Work out the finished part from the listing and answer in its coordinate system (mm). A direction names the side the tool comes from. Coordinates: 2 decimals unless noted, no trailing zeros. Use a Markdown table: item, result.
from build123d import *

# Parameters (mm, degrees)
BOSS_EXTRUDE1_DEPTH = 30
CHAMFER1_SIZE       = 13.5
FILLET1_R           = 50
FILLET2_R           = 50
SHELL1_T            = -5
CUT_EXTRUDE1_REACH  = 183.384
SKETCH5_W           = 85.5
SKETCH5_H           = 65.5
CUT_EXTRUDE2_DEPTH  = 2
SKETCH6_R           = 10.1203125
CUT_EXTRUDE3_DEPTH  = 1.488
CUT_EXTRUDE4_START  = -1.488
SKETCH7_R           = 10.1203125
CUT_EXTRUDE4_DEPTH  = 1.488
CUT_EXTRUDE5_REACH  = 198.109
SKETCH8_R           = 7.9375
BOSS_EXTRUDE2_START = -25
BOSS_EXTRUDE2_DEPTH = 22.5
CUT_EXTRUDE6_START  = -2.5
CUT_EXTRUDE6_DEPTH  = 5
SKETCH11_R          = 2.1
CUT_EXTRUDE7_DEPTH  = 155.677082983
CUT_EXTRUDE8_REACH  = 210.327
SKETCH12_R          = 8.1


with BuildPart() as part:
    # Sketch3 → Boss-Extrude1 (new body)
    with BuildSketch(Plane(origin=(0, 0, 0), x_dir=(1, 0, 0), z_dir=(0, 1, 0))):
        Polygon((80, 0), (80, -100), (30, -130), (-30, -130), (-80, -100), (-80, 0), (-30, 30), (30, 30), align=None)
    extrude(amount=BOSS_EXTRUDE1_DEPTH)

    # Chamfer1
    chamfer1_edges = [part.edges().sort_by_distance(p)[0] for p in [
        (-55, 30, 115),
        (0, 30, 130),
        (55, 30, 115),
    ]]
    chamfer(chamfer1_edges, length=CHAMFER1_SIZE)

    # Fillet1
    # the kernel refuses this fillet: 50 mm, written as the material it takes off along each edge
    with BuildSketch(Plane(origin=(30, -34.622995619, 130), x_dir=(0.857492925712544, 0, -0.5144957554275268), z_dir=(0, 1, 0)), Plane(origin=(-30, -34.622995619, 130), x_dir=(1, 0, 0), z_dir=(0, 1, 0))) as fillet1_piece_1:
        with BuildLine():
            CenterArc((FILLET1_R * 0.276983964948, FILLET1_R), FILLET1_R, 239.036243468, 30.963756532)
            Line((-FILLET1_R * 0.237511790479, FILLET1_R * 0.142507074287), (0, 0))
            Line((0, 0), (FILLET1_R * 0.276983964948, 0))
        make_face()
    extrude(amount=85.745991237, mode=Mode.SUBTRACT)
    with BuildSketch(Plane(origin=(-80, -39.074271729, 164.810181009), x_dir=(0, -0.759125277171481, -0.6509445549041194), z_dir=(0, 0.6509445549041194, -0.759125277171481))) as fillet1_piece_2:
        with BuildLine():
            CenterArc((FILLET1_R * 0.682998529574, -FILLET1_R), FILLET1_R, 90, 68.666037253)
            Line((-FILLET1_R * 0.248477212904, -FILLET1_R * 0.636196562446), (0, 0))
            Line((0, 0), (FILLET1_R * 0.682998529574, 0))
        make_face()
    extrude(amount=191.488725913, mode=Mode.SUBTRACT)
    with BuildSketch(Plane(origin=(80, -39.074271729, 164.810181009), x_dir=(0, -0.759125277171481, -0.6509445549041195), z_dir=(0, 0.6509445549041195, -0.759125277171481))) as fillet1_piece_3:
        with BuildLine():
            CenterArc((FILLET1_R * 0.682998529574, FILLET1_R), FILLET1_R, 201.333962747, 68.666037253)
            Line((-FILLET1_R * 0.248477212904, FILLET1_R * 0.636196562446), (0, 0))
            Line((0, 0), (FILLET1_R * 0.682998529574, 0))
        make_face()
    extrude(amount=191.488725913, mode=Mode.SUBTRACT)
    with BuildSketch(Plane(origin=(34.617865704, -0.171960433, 146.671960433), x_dir=(0.9114297192816029, -0.13590975982943138, -0.3883611772478869), z_dir=(-0.19220542560964893, 0.6939225729021263, -0.6939225729021263)), Plane(origin=(-34.617865704, -0.171960433, 146.671960433), x_dir=(0.9813547138350198, -0.13590975982942916, 0.13590975982942954), z_dir=(0.19220542560964907, 0.6939225729021263, -0.6939225729021263))) as fillet1_piece_4:
        with BuildLine():
            CenterArc((FILLET1_R * 0.19220542561, FILLET1_R), FILLET1_R, 248.24024707, 21.75975293)
            Line((-FILLET1_R * 0.178510109177, FILLET1_R * 0.0712535371437), (0, 0))
            Line((0, 0), (FILLET1_R * 0.19220542561, 0))
        make_face()
    extrude(amount=67.505976453, mode=Mode.SUBTRACT)

    # Fillet2
    fillet2_edges = [part.edges().sort_by_distance(p)[0] for p in [
        (30, 15, -30),
        (-30, 15, -30),
    ]]
    fillet(fillet2_edges, radius=FILLET2_R)

    # Shell1
    shell1_openings = [part.faces().sort_by_distance(p)[0] for p in [
        (0, 30, 41.507073617),
    ]]
    offset(amount=SHELL1_T, openings=shell1_openings)

    # Sketch4 → Cut-Extrude1 (cut, up to next)
    with BuildSketch(Plane.XY.offset(130), mode=Mode.PRIVATE) as cut_extrude1_sk1:
        Polygon((10.55, 13.832263561), (10.55, 8.567736439), (6.776999518, 6), (-10.55, 6), (-10.55, 16.4), (6.776999518, 16.4), align=None)
    cut_extrude1_tool1 = extrude(cut_extrude1_sk1.sketch, amount=-CUT_EXTRUDE1_REACH, mode=Mode.PRIVATE) & part.part
    add(cut_extrude1_tool1.solids().sort_by_distance((-0.429196, 11.2, 130))[0], mode=Mode.SUBTRACT)

    # Sketch5 → Cut-Extrude2 (cut)
    with BuildSketch(Plane(origin=(0, 5, 0), x_dir=(1, 0, 0), z_dir=(0, 1, 0))):
        with Locations((-7.25, -42.75)):
            Rectangle(SKETCH5_W, SKETCH5_H)
    extrude(amount=-CUT_EXTRUDE2_DEPTH, mode=Mode.SUBTRACT)

    # Sketch6 → Cut-Extrude3 (cut)
    with BuildSketch(Plane(origin=(21.176470588, 0, -35.294117647), x_dir=(-0.8574929257125442, 0, -0.5144957554275265), z_dir=(0.5144957554275265, 0, -0.8574929257125442))):
        with Locations((-39.259425856, 15.1203125)):
            Circle(SKETCH6_R)
    cut_extrude3 = extrude(amount=-CUT_EXTRUDE3_DEPTH, mode=Mode.SUBTRACT)

    # Sketch7 → Cut-Extrude4 (cut)
    with BuildSketch(Plane(origin=(18.603991811, 0, -31.006653018), x_dir=(0.8574929257125442, 0, 0.5144957554275265), z_dir=(-0.5144957554275265, 0, 0.8574929257125442)).offset(CUT_EXTRUDE4_START)):
        with Locations(Location((39.259425856, 15.1203125, 0), (0, 0, 180))):
            Circle(SKETCH7_R)
    cut_extrude4 = extrude(amount=CUT_EXTRUDE4_DEPTH, mode=Mode.SUBTRACT)

    # Sketch8 → Cut-Extrude5 (cut, up to next)
    with BuildSketch(Plane(origin=(21.176470588, 0, -35.294117647), x_dir=(-0.8574929257125442, 0, -0.5144957554275265), z_dir=(0.5144957554275265, 0, -0.8574929257125442)), mode=Mode.PRIVATE) as cut_extrude5_sk1:
        with Locations((-39.259425856, 15.1203125)):
            Circle(SKETCH8_R)
    cut_extrude5_tool1 = extrude(cut_extrude5_sk1.sketch, amount=-CUT_EXTRUDE5_REACH, mode=Mode.PRIVATE) & part.part
    cut_extrude5 = cut_extrude5_tool1.solids().sort_by_distance((54.841151, 15.120313, -15.09531))[0]
    add(cut_extrude5, mode=Mode.SUBTRACT)

    # Mirror1: Cut-Extrude3, Cut-Extrude4, Cut-Extrude5 across plane
    add(cut_extrude3.mirror(Plane(origin=(0, 0, 0), x_dir=(0, 0, 1), z_dir=(1, 0, 0))), mode=Mode.SUBTRACT)
    add(cut_extrude4.mirror(Plane(origin=(0, 0, 0), x_dir=(0, 0, 1), z_dir=(1, 0, 0))), mode=Mode.SUBTRACT)
    add(cut_extrude5.mirror(Plane(origin=(0, 0, 0), x_dir=(0, 0, 1), z_dir=(1, 0, 0))), mode=Mode.SUBTRACT)

    # Sketch9 → Boss-Extrude2 (add)
    with BuildSketch(Plane(origin=(0, 30, 0), x_dir=(1, 0, 0), z_dir=(0, 1, 0)).offset(BOSS_EXTRUDE2_START)):
        with BuildLine():
            Line((-75, -2.830951895), (-66.425070743, 2.314005659))
            Line((-66.425070743, 2.314005659), (-62.074071209, -0.149488415))
            ThreePointArc((-62.074071209, -0.149488415), (-58.789057061, -12.009431821), (-70.649000466, -15.29444597))
            Line((-70.649000466, -15.29444597), (-75, -12.830951895))
            Line((-75, -12.830951895), (-75, -2.830951895))
        make_face()
    boss_extrude2 = extrude(amount=BOSS_EXTRUDE2_DEPTH)

    # Sketch10 → Cut-Extrude6 (cut)
    with BuildSketch(Plane(origin=(0, 30, 0), x_dir=(1, 0, 0), z_dir=(0, 1, 0)).offset(CUT_EXTRUDE6_START)):
        Polygon((-62.361535838, -5.412566116), (-66.361535838, -3.103165039), (-70.361535838, -5.412566116), (-70.361535838, -10.031368269), (-66.361535838, -12.340769346), (-62.361535838, -10.031368269), align=None)
    cut_extrude6 = extrude(amount=-CUT_EXTRUDE6_DEPTH, mode=Mode.SUBTRACT)

    # Mirror2: Boss-Extrude2, Cut-Extrude6 across plane
    add(boss_extrude2.mirror(Plane(origin=(0, 0, 0), x_dir=(0, 0, 1), z_dir=(1, 0, 0))))
    add(cut_extrude6.mirror(Plane(origin=(0, 0, 0), x_dir=(0, 0, 1), z_dir=(1, 0, 0))), mode=Mode.SUBTRACT)

    # Sketch11 → Cut-Extrude7 (cut, through all)
    with BuildSketch(Plane(origin=(0, 5, 0), x_dir=(1, 0, 0), z_dir=(0, 1, 0))):
        with Locations(Location((-27.25, -95.5, 0), (0, 0, 270))):
            Circle(SKETCH11_R)
        with Locations(Location((-20, 19, 0), (0, 0, 270))):
            Circle(SKETCH11_R)
    cut_extrude7 = extrude(amount=-CUT_EXTRUDE7_DEPTH, mode=Mode.SUBTRACT)

    # Mirror3: Cut-Extrude7 across plane
    add(cut_extrude7.mirror(Plane(origin=(0, 0, 0), x_dir=(0, 0, 1), z_dir=(1, 0, 0))), mode=Mode.SUBTRACT)

    # Sketch12 → Cut-Extrude8 (cut, up to next)
    with BuildSketch(Plane(origin=(80, 0, 0), x_dir=(0, 0, -1), z_dir=(1, 0, 0)), mode=Mode.PRIVATE) as cut_extrude8_sk1:
        with Locations((-32.830951895, 16.25)):
            Circle(SKETCH12_R)
    cut_extrude8_tool1 = extrude(cut_extrude8_sk1.sketch, amount=-CUT_EXTRUDE8_REACH, mode=Mode.PRIVATE) & part.part
    add(cut_extrude8_tool1.solids().sort_by_distance((80, 16.25, 32.830952))[0], mode=Mode.SUBTRACT)


solid = part.part
Q1. Consider line 1 (X direction, y = 6.5, z = 39.5); line 2 (Z direction, x = 27.25, y = 3.3); line 3 (X direction, y = 18.5, z = 14). Determine where each line is inside the solid, lowest interval first. Write a range as [from, to].
Solved:
| item | result |
|---|---|
| line 1 | [-80, -75], [75, 80] |
| line 2 | [-28.75, 10], [75.5, 93.4], [97.6, 128.75] |
| line 3 | [-80, -75], [-72.94, -60.34], [60.34, 72.94], [75, 80] |
Q2. Given pin 1 Ø2.5 at (x, z) = (-3, 128.5) entering from +Y; pin 2 Ø1.5 at (y, z) = (12, 126.5) entering from -X; pin 3 Ø5 at (x, z) = (20, -19) entering from +Y; pin 4 Ø5 at (x, z) = (55, -11) entering from -Y, each flat-ended and moving along its own axis, determine where each tip first touches the part or whether it passes through.
Solved:
| item | result |
|---|---|
| pin 1 | y = 19.25 |
| pin 2 | x = -36.32 |
| pin 3 | y = 5 |
| pin 4 | y = 0 |
Q3. For faces 4 (the flat face through (-2, 6, 128)), 5 (the cylindrical face through (-74.854, 16.573, 81.392)), 6 (the flat face through (-68.33, 25.04, 4.24)), 7 (the cylindrical face through (19.369, 2.535, -16.997)), 8 (the cylindrical face through (25.908, 22.64, 115.676)), determine the directions among +Z, -Z, +X, -X, +Y, -Y from which every point of the face is accessible in a straight line to the end or side of a thin tool.
Solved:
| item | result |
|---|---|
| face 4 | +Z |
| face 5 | +Z, -X, +Y |
| face 6 | +Y |
| face 7 | +Y, -Y |
| face 8 | none |
Q4. Section A-A on y = 10.5 is taken. State how many separate pieces and enclosed holes the cut face has, and give its area (3 significant figures).
Solved:
| item | result |
|---|---|
| separate pieces | 4 |
| enclosed holes | 0 |
| area | 2,820 mm² |
Q5. Determine the mould class of faces 1 (the cylindrical face through (27.519, 23.723, 121.541)), 2 (the cylindrical face through (58.697, 16.093, 11.842)), 3 (the flat face through (1, 0, 49)) for opening direction X: pulls with the +X half, pulls with the -X half, needs draft (parallel to the pull), parting line crosses it, or undercut.
Solved:
| item | result |
|---|---|
| face 1 | pulls with the +X half |
| face 2 | undercut |
| face 3 | needs draft |
